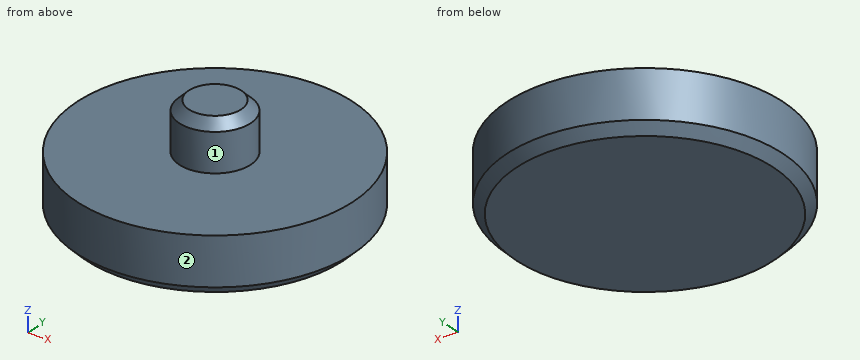
```python
from build123d import *

# Parameters (mm, degrees)
F0_R     = 29
F1_DEPTH = 12
F2_R     = 7.5
F3_DEPTH = 10
F4_SIZE  = 2
F5_SIZE  = 2


with BuildPart() as f1:
    # F0 (on Top) → F1 (new body)
    with BuildSketch(Plane.XY):
        Circle(F0_R)
    extrude(amount=F1_DEPTH)

    # F2 (on face) → F3 (join)
    with BuildSketch(Plane.XY.offset(12)):
        Circle(F2_R)
    extrude(amount=F3_DEPTH)

    # F4
    f4_edges = [f1.edges().sort_by_distance(p)[0] for p in [
        (-7.5, 0, 22),
    ]]
    chamfer(f4_edges, length=F4_SIZE)

    # F5
    f5_edges = [f1.edges().sort_by_distance(p)[0] for p in [
        (-29, 0, 0),
    ]]
    chamfer(f5_edges, length=F5_SIZE)


solid = f1.part
```
Read the model definition and answer for the solid it produces. Units are mm, in the model's axes. Face numbers are marked on the shaded views. A direction names the side the tool comes from. Give positions to 0.01 mm unless a question says otherwise; leave off trailing zeros. Write each loop counter-clockwise with the first axis right and the second up, starting at its lowest first coordinate (ties: lowest second). Pieces come first, ordered by that corner, then holes. Notation, with made-up numbers: (-23, 60.25) -> (3, 60.25) arc R32 cw to (3, 95.25) -> close; hole circle Ø1 at (81.25, 52). An arc over 180 degrees is marked (long way). Answer as a JSON object with one key per item and string values.
1) Section A-A on y = 0 is taken. Write down the section's boundary in (x, z), then the cut area to 3 significant figures.
Findings below:
{"outline": "(-29, 2) -> (-27, 0) -> (27, 0) -> (29, 2) -> (29, 12) -> (7.5, 12) -> (7.5, 20) -> (5.5, 22) -> (-5.5, 22) -> (-7.5, 20) -> (-7.5, 12) -> (-29, 12) -> close", "area": "838 mm^2"}
2) Straight lines are drawn through the part: probe 1 along Z at (x, y) = (12.5, 12.5); probe 2 along X at (y, z) = (0.5, 4.75); probe 3 along Y at (x, z) = (-20, 2). For each, find the intervals that lie inside material, in ascending order. Write a range as from..to.
Findings below:
{"probe 1": "z = 0..12", "probe 2": "x = -29..29", "probe 3": "y = -21..21"}
3) Flat-ended cylindrical pins translate along their axes: pin 1 Ø12 at (y, z) = (15.5, 12) entering from +X; pin 2 Ø3 at (x, z) = (-5, 14) entering from +Y; pin 3 Ø3 at (x, z) = (8, 11) entering from -Y. Find the tip coordinate at first contact, or state that the pin passes through.
Findings below:
{"pin 1": "stops at x = 27.4", "pin 2": "stops at y = 6.63", "pin 3": "stops at y = -28.26"}
4) Section C-C on z = 16.75 is taken. Write down the section's boundary in (x, y), then the cut area to 3 significant figures.
Findings below:
{"outline": "circle Ø15 at (0, 0)", "area": "177 mm^2"}
5) Section D-D on z = 7.25 is taken. Write down the section's boundary in (x, y), then the cut area to 3 significant figures.
Findings below:
{"outline": "circle Ø58 at (0, 0)", "area": "2,640 mm^2"}
6) A tool of negligible diameter and unlimited length cuts with its end or side. For the marked faces 1 and 2, from which of +Z, -Z, +X, -X, +Y, -Y can it reach the whole face along a straight path? Write none if from no direction.
Findings below:
{"face 1": "+Z", "face 2": "+Z, -Z"}
